from build123d import *

# Parameters (mm, degrees)
SKETCH1_W               = 13
SKETCH1_H               = 13
BOSS_EXTRUDE1_DEPTH     = 10
SKETCH2_R               = 9.3
BOSS_EXTRUDE2_DEPTH     = 34
SKETCH3_W               = 32
SKETCH3_H               = 10
SKETCH3_W_2             = 7.2
SKETCH3_H_2             = 4
BOSS_EXTRUDE3_DEPTH     = 3
CUT_EXTRUDE1_DEPTH      = 42.817938734
CUT_EXTRUDE1_DEPTH_BACK = 42.817938734
SKETCH5_W               = 7.2
SKETCH5_H               = 4
CUT_EXTRUDE2_DEPTH      = 25
CHAMFER1_SIZE           = 7
CHAMFER1_SIZE_2         = 4.041451884


with BuildPart() as part:
    # Sketch1 → Boss-Extrude1 (new body)
    with BuildSketch(Plane(origin=(0, 0, 0), x_dir=(1, 0, 0), z_dir=(0, 1, 0))):
        with Locations((0, -0.046937875)):
            Rectangle(SKETCH1_W, SKETCH1_H)
    extrude(amount=BOSS_EXTRUDE1_DEPTH)

    # Sketch2 → Boss-Extrude2 (add)
    with BuildSketch(Plane.XZ):
        with Locations(Location((0, 0, 0), (0, 0, 270))):
            Circle(SKETCH2_R)
    extrude(amount=BOSS_EXTRUDE2_DEPTH)

    # Sketch3 → Boss-Extrude3 (add)
    with BuildSketch(Plane.XZ.offset(34)):
        Rectangle(SKETCH3_W, SKETCH3_H)
        with Locations((-9.4, 0)):
            Rectangle(SKETCH3_W_2, SKETCH3_H_2, mode=Mode.SUBTRACT)
        with Locations((9.4, 0)):
            Rectangle(SKETCH3_W_2, SKETCH3_H_2, mode=Mode.SUBTRACT)
    extrude(amount=-BOSS_EXTRUDE3_DEPTH)

    # Sketch4 → Cut-Extrude1 (cut, two sides: drawn at the far end of the back side and taken through both)
    with BuildSketch(Plane.ZY.offset(6.5).offset(-CUT_EXTRUDE1_DEPTH_BACK)):
        Polygon((-3.953062125, 0), (4.046937875, 0), (0.046937875, 6.92820323), align=None)
    extrude(amount=CUT_EXTRUDE1_DEPTH + CUT_EXTRUDE1_DEPTH_BACK, mode=Mode.SUBTRACT)

    # Sketch5 → Cut-Extrude2 (cut)
    with BuildSketch(Plane.XZ.offset(34)):
        with Locations((-9.4, 0)):
            Rectangle(SKETCH5_W, SKETCH5_H)
        with Locations((9.4, 0)):
            Rectangle(SKETCH5_W, SKETCH5_H)
    extrude(amount=-CUT_EXTRUDE2_DEPTH, mode=Mode.SUBTRACT)

    # Chamfer1
    # the kernel refuses this chamfer: 7, 4.041451884 mm, written as the material it adds along each edge
    with BuildSketch(Plane(origin=(-5.8, -9, -20.109600283), x_dir=(0.01932676561270078, -0.9998132206222078, 0), z_dir=(0, 0, 1))) as chamfer1_piece_1_section:
        Polygon((CHAMFER1_SIZE * 0.999813220622, -CHAMFER1_SIZE * 0.0193267656127), (-CHAMFER1_SIZE_2 * 0.0193267656143, -CHAMFER1_SIZE_2 * 0.999813220703), (0, 0), align=None)
    chamfer1_piece_1 = extrude(amount=40.219200565, mode=Mode.PRIVATE)
    chamfer1_piece_1 = chamfer1_piece_1 & Plane(origin=(0, -11.718976522, 0), x_dir=(0, 0, -1), z_dir=(0, 1, 0)) * Cylinder(9.3, 109, mode=Mode.PRIVATE)
    add(chamfer1_piece_1)
    with BuildSketch(Plane(origin=(5.8, -9, 20.109600283), x_dir=(-0.01932676561270078, -0.9998132206222078, 0), z_dir=(0, 0, -1))) as chamfer1_piece_2_section:
        Polygon((CHAMFER1_SIZE * 0.999813220622, -CHAMFER1_SIZE * 0.0193267656127), (-CHAMFER1_SIZE_2 * 0.0193267656143, -CHAMFER1_SIZE_2 * 0.999813220703), (0, 0), align=None)
    chamfer1_piece_2 = extrude(amount=40.219200565, mode=Mode.PRIVATE)
    chamfer1_piece_2 = chamfer1_piece_2 & Plane(origin=(0, -11.718976523, 0), x_dir=(0, 0, -1), z_dir=(0, 1, 0)) * Cylinder(9.3, 109, mode=Mode.PRIVATE)
    add(chamfer1_piece_2)


solid = part.part
The listing builds one solid part. Answer for the finished solid, in the listing's coordinates (mm). A direction names the side the tool comes from. Give positions to 0.01 mm unless a question says otherwise; leave off trailing zeros. Loops run counter-clockwise (first coordinate to the right, second up) from the corner with the lowest first, then second, coordinate; pieces in that order, holes last. Notation, with made-up numbers: (61.25, 67) - (101.25, 67) arc R23 cw to (101.25, 104) - close; hole circle Ø8 at (-25.5, -28.75). An arc over 180 degrees is marked (long way). Answer as a JSON object with one key per item and string values.
1. A cutting plane is placed at C-C (x = -11). Write down the section's boundary in (y, z).
Determined:
{"outline": "(-34, -5) - (-31, -5) - (-31, -2) - (-34, -2) - close; (-34, 2) - (-31, 2) - (-31, 5) - (-34, 5) - close"}
2. Flat-ended cylindrical pins translate along their axes: pin 1 Ø5 at (y, z) = (6, -2) entering from +X; pin 2 Ø8 at (x, y) = (5.5, 2) entering from -Z; pin 3 Ø8 at (x, y) = (-10, -19.5) entering from +Z. Find the tip coordinate at first contact, or state that the pin passes through.
Determined:
{"pin 1": "x = 6.5", "pin 2": "z = -9.07", "pin 3": "z = 7.11"}
3. A cutting plane is placed at B-B (y = 2). Write down the section's boundary in (x, z), then the cut area to 3 significant figures.
Determined:
{"outline": "(-6.5, -6.45) - (6.5, -6.45) - (6.5, -2.8) - (-6.5, -2.8) - close; (-6.5, 2.89) - (6.5, 2.89) - (6.5, 6.55) - (-6.5, 6.55) - close", "area": "95.0 mm²"}
4. A cutting plane is placed at D-D (z = -2.5). Write down the section's boundary in (x, y), then the cut area to 3 significant figures.
Determined:
{"outline": "(-16, -34) - (16, -34) - (16, -31) - (8.96, -31) - (8.96, 0) - (-8.96, 0) - (-8.96, -31) - (-16, -31) - close; (-6.5, 2.52) - (6.5, 2.52) - (6.5, 10) - (-6.5, 10) - close", "area": "749 mm²"}
5. Find the intervals of material crossed by L1, parallel to Y at x = 9.5, z = 2.25; L2, parallel to Y at x = 8, z = -2.5; L3, parallel to X at y = -24.5, z = 0, in increasing order. Write a range as [from, to].
Determined:
{"L1": "[-34, -31]", "L2": "[-34, 0]", "L3": "[-5.8, 5.8]"}
6. For a pull along X with two mould halves and no side action, classify faces 4 (the flat face through (0, 5, -6.453)), 5 (the flat face through (-13, -33, 0)), 6 (the flat face through (-7.526, -13.011, -0.028)) as pulls with the +X half, pulls with the -X half, needs draft (parallel to the pull), parting line crosses it, or undercut.
Determined:
{"face 4": "needs draft", "face 5": "undercut", "face 6": "pulls with the -X half"}
7. For faces 1 (the flat face through (-8, -25, -2)), 2 (the flat face through (13, -33, 0)), 3 (the flat face through (0, 5, 6.547)), determine the directions among +Z, -Z, +X, -X, +Y, -Y from which every point of the face is accessible in a straight line to the end or side of a thin tool.
Determined:
{"face 1": "-Y", "face 2": "+Y, -Y", "face 3": "+Z, +X, -X, +Y"}
8. A cutting plane is placed at A-A (x = 0). Write down the section's boundary in (y, z).
Determined:
{"outline": "(-34, -9.3) - (0, -9.3) - (0, -6.45) - (10, -6.45) - (10, 6.55) - (0, 6.55) - (0, 9.3) - (-34, 9.3) - close; hole (0, -3.95) - (6.93, 0.05) - (0, 4.05) - close"}
